Autodesk Inventor part; units mm, degrees
ref_plane "YZ Plane" through (0, 0, 0) normal (1, 0, 0) x (0, 1, 0)
ref_plane "XZ Plane" through (0, 0, 0) normal (0, 1, 0) x (-1, 0, 0)
ref_plane "XY Plane" through (0, 0, 0) normal (0, 0, 1) x (1, 0, 0)
sketch "Sketch1" plane through (0, 0, 0) normal (0, 0, 1) x (1, 0, 0)
  circle A0 centre (0, 0) radius 2.0955
  circle A1 centre (0, 12.7) radius 2.0955
  circle A2 centre (19.05, 6.35) radius 2.1209
  circle A3 centre (38.1, 12.7) radius 2.0955
  circle A4 centre (25.4, -12.7) radius 2.0955
  arc A5 (-6.3002, 0.7937) -> (-2.8398, -5.6796) centre (0, 0) ccw
  arc A6 (1.506, 17.2181) -> (-4.7251, 13.2953) centre (0, 12.7) ccw
  arc A7 (42.896, 8.5381) -> (36.3, 18.7895) centre (38.1, 12.7) ccw
  arc A8 (22.5602, -18.3796) -> (31.7002, -13.4938) centre (25.4, -12.7) ccw
  circle A9 centre (25.4, 0) radius 5.461
  line L0 (9.6793, 14.4937) -> (1.506, 17.2181)
  line L1 (36.3, 18.7895) -> (21.1035, 14.2975)
  arc A10 (9.6793, 14.4937) -> (21.1035, 14.2975) centre (15.7034, 32.5661) ccw
  arc A11 (42.896, 8.5381) -> (31.6071, -14.0397) centre (81.2637, -24.7569) ccw
  line L2 (-4.7251, 13.2953) -> (-6.3002, 0.7937)
  line L3 (-2.8398, -5.6796) -> (22.5602, -18.3796)
  point P0 (40.6465, 18.517)
  point P1 (44.45, 12.7)
  dimension "d0" = 4.191
  dimension "d1" = 4.191
  dimension "d2" = 4.2418
  dimension "d3" = 4.191
  dimension "d4" = 4.191
  dimension "d5" = 12.7
  dimension "d9" = 10.922
  dimension "d10" = 19.05
  dimension "d16" = 6.35
extrude "Extrusion1" add sketch "Sketch1" along normal blind 1.5875
equation "\"BendRadius\" = Thickness"
equation "\"BendReliefWidth\" = Thickness"
equation "\"BendReliefDepth\" = 0.5 * Thickness"
equation "\"CornerReliefSize\" = 4 * Thickness"
equation "\"MinimumRemnant\" = 2 * Thickness"
equation "\"TransitionRadius\" = BendRadius"
equation "\"JacobiRadiusSize\" = BendRadius"
equation "\"GapSize\" = Thickness"
properties part number "gearbox_gusset" material "Acetal Resin, White"
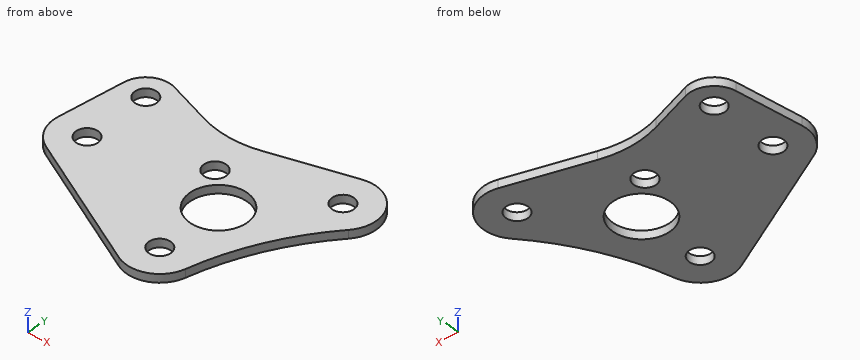
Design review of the part built by this model. Coordinates are the model's own, in mm. Round coordinates to 2 decimals unless told otherwise and drop trailing zeros. Write each loop counter-clockwise with the first axis right and the second up, starting at its lowest first coordinate (ties: lowest second). Pieces come first, ordered by that corner, then holes. Notation, with made-up numbers: (29, -1.5) -> (64, -1.5) arc R14 ccw to (64, 25.5) -> close; hole circle Ø3 at (6, 66). An arc over 180 degrees is marked (long way). One line per item, written item: value. Start each with the question number.
Q1. Add section C-C (y = -13.5). Give the boundary of the cut face in (x, z), then the cut area to 3 significant figures.
Q2. Add section A-A (z = 0.7). Give the boundary of the cut face in (x, y), then the cut area to 3 significant figures.
Q3. To check wall thickness, follow probe 1 along Y at (x, z) = (25.4, 1.2); probe 2 along Y at (x, z) = (0.5, 0.15); probe 3 along X at (y, z) = (1, 0.55). State the ranges of each line that lie inside material, in increasing order.
Q4. Insertion check: P1, Ø5, axis at x = -0.5, y = -5, coming from the -Z side; P2, Ø3.5, axis at x = 0, y = 12.7, coming from the -Z side. Each pin has a flat end and moves straight along its axis. Give the tip position at first contact, or say it passes through.
Q5. Add section D-D (x = 0). Give the boundary of the cut face in (y, z), then the cut area to 3 significant figures.
Q6. Add section B-B (x = 19.05). Give the boundary of the cut face in (y, z), then the cut area to 3 significant figures.
Response:
1. outline: (12.8, 0) -> (23.46, 0) -> (23.46, 1.59) -> (12.8, 1.59) -> close; (27.34, 0) -> (31.73, 0) -> (31.73, 1.59) -> (27.34, 1.59) -> close
1. area: 23.9 mm^2
2. outline: (-6.3, 0.79) arc R6.35 ccw to (-2.84, -5.68) -> (22.56, -18.38) arc R6.35 ccw to (31.61, -14.04) arc R50.8 cw to (42.9, 8.54) arc R6.35 ccw to (36.3, 18.79) -> (21.1, 14.3) arc R19.05 cw to (9.68, 14.49) -> (1.51, 17.22) arc R4.76 ccw to (-4.73, 13.3) -> close; hole circle Ø4.19 at (0, 0); hole circle Ø4.19 at (0, 12.7); hole circle Ø4.24 at (19.05, 6.35); hole circle Ø10.92 at (25.4, 0); hole circle Ø4.19 at (25.4, -12.7); hole circle Ø4.19 at (38.1, 12.7)
2. area: 1,110 mm^2
3. probe 1: y = -19.05 to -14.8, -10.6 to -5.46, 5.46 to 15.57
3. probe 2: y = -7.35 to -2.03, 2.03 to 10.67, 14.73 to 17.44
3. probe 3: x = -6.27 to -1.84, 1.84 to 20.03, 30.77 to 37.48
4. P1: stops at z = 0
4. P2: passes through
5. outline: (-7.1, 0) -> (-2.1, 0) -> (-2.1, 1.59) -> (-7.1, 1.59) -> close; (2.1, 0) -> (10.6, 0) -> (10.6, 1.59) -> (2.1, 1.59) -> close; (14.8, 0) -> (17.46, 0) -> (17.46, 1.59) -> (14.8, 1.59) -> close
5. area: 25.7 mm^2
6. outline: (-16.62, 0) -> (4.23, 0) -> (4.23, 1.59) -> (-16.62, 1.59) -> close; (8.47, 0) -> (13.81, 0) -> (13.81, 1.59) -> (8.47, 1.59) -> close
6. area: 41.6 mm^2
